```python
from build123d import *

# Parameters (mm, degrees)
F0_W     = 42.3
F0_H     = 42.3
F1_DEPTH = 48
F2_R     = 1.5
F3_DEPTH = 4.5
F4_R     = 11
F5_DEPTH = 2
F6_SIZE  = 5
F7_R     = 2.5
F8_DEPTH = 19
F9_R     = 0.5
F10_R    = 3


with BuildPart() as f1:
    # F0 (on Front) → F1 (new body)
    with BuildSketch(Plane.XZ):
        Rectangle(F0_W, F0_H)
    extrude(amount=F1_DEPTH)

    # F2 (on face) → F3 (cut)
    with BuildSketch(Plane.XZ.offset(48)):
        with Locations((-15.5, 15.5)):
            Circle(F2_R)
        with Locations((-15.5, -15.5)):
            Circle(F2_R)
        with Locations((15.5, -15.5)):
            Circle(F2_R)
        with Locations((15.5, 15.5)):
            Circle(F2_R)
    extrude(amount=-F3_DEPTH, mode=Mode.SUBTRACT)

    # F4 (on face) → F5 (join)
    with BuildSketch(Plane.XZ.offset(48)):
        Circle(F4_R)
    extrude(amount=F5_DEPTH)

    # F6
    f6_edges = [f1.edges().sort_by_distance(p)[0] for p in [
        (21.15, -24, 21.15),
        (-21.15, -24, 21.15),
        (-21.15, -24, -21.15),
        (21.15, -24, -21.15),
    ]]
    chamfer(f6_edges, length=F6_SIZE)

    # F7 (on face) → F8 (join)
    with BuildSketch(Plane.XZ.offset(50)):
        Circle(F7_R)
    extrude(amount=F8_DEPTH)

    # F9
    f9_edges = [f1.edges().sort_by_distance(p)[0] for p in [
        (-2.5, -69, 0),
    ]]
    fillet(f9_edges, radius=F9_R)

    # F10
    f10_edges = [f1.edges().sort_by_distance(p)[0] for p in [
        (16.15, -24, -21.15),
        (21.15, -24, -16.15),
        (-16.15, -24, -21.15),
        (-21.15, -24, -16.15),
        (21.15, -24, 16.15),
        (16.15, -24, 21.15),
        (-16.15, -24, 21.15),
        (-21.15, -24, 16.15),
    ]]
    fillet(f10_edges, radius=F10_R)


solid = f1.part
```
Design review of the part built by this model. Coordinates are the model's own, in mm. A direction names the side the tool comes from. Coordinates: 2 decimals unless noted, no trailing zeros. Write each loop counter-clockwise with the first axis right and the second up, starting at its lowest first coordinate (ties: lowest second). Pieces come first, ordered by that corner, then holes.
1) Mouldability with a two-part tool opening along Z and no side actions: class faces 1 (the cylindrical face through (-16.071, -24.336, 20.915)), 2 (the flat face through (15, -43.5, -15)), 3 (the flat face through (-3, -50, 0)), 4 (the cylindrical face through (-20.93, -24.34, -16.04)) as +Z half, -Z half, draft (parallel to the pull), parting line (faces both ways), or undercut.
2) Add section D-D (x = -4.5). Write out the cut boundary in (y, z), plus the area to 3 significant figures.
3) Insertion check: pin 1 (1 mm diameter, centred on x = 10.5, z = 3, fed in from -Y); pin 2 (0.9 mm diameter, centred on x = 16, z = -16, fed in from -Y); pin 3 (2.5 mm diameter, centred on x = -15, z = 16, fed in from -Y). Each pin has a flat end and moves straight along its axis. Give the tip position at first contact, or say it passes through.
4) Add section C-C (z = 5). Write out the cut boundary in (x, y).
5) Machinability: for faces 5 (the cylindrical face through (-17, -45.78, -15.43)), 6 (the cylindrical face through (-16.071, -24.336, -20.915)), which of the approach directions +Z, -Z, +X, -X, +Y, -Y give a long, thin tool a straight path to every point of the face, cutting with its end or side? Answer none if there is none.
6) Add section A-A (y = -14). Write out the cut boundary in (x, z).
7) Add section B-B (x = 0). Write out the cut boundary in (y, z).
8) To check wall thickness, follow L1, parallel to Z at x = -15.5, y = -47.1; L2, parallel to Z at x = 15, y = -46. State the ranges of each line that lie inside material, in increasing order.
Check result:
1. face 1: +Z half
1. face 2: undercut
1. face 3: draft
1. face 4: -Z half
2. outline: (-50, -10.04) - (-48, -10.04) - (-48, -21.15) - (0, -21.15) - (0, 21.15) - (-48, 21.15) - (-48, 10.04) - (-50, 10.04) - close
2. area: 2,070 mm2
3. pin 1: stops at y = -50
3. pin 2: stops at y = -43.5
3. pin 3: stops at y = -48
4. outline: (-21.15, -48) - (-9.8, -48) - (-9.8, -50) - (9.8, -50) - (9.8, -48) - (21.15, -48) - (21.15, 0) - (-21.15, 0) - close
5. face 5: -Y
5. face 6: -Z, -X, +Y, -Y
6. outline: (-21.15, -14.91) arc R3 ccw to (-20.27, -17.03) - (-17.03, -20.27) arc R3 ccw to (-14.91, -21.15) - (14.91, -21.15) arc R3 ccw to (17.03, -20.27) - (20.27, -17.03) arc R3 ccw to (21.15, -14.91) - (21.15, 14.91) arc R3 ccw to (20.27, 17.03) - (17.03, 20.27) arc R3 ccw to (14.91, 21.15) - (-14.91, 21.15) arc R3 ccw to (-17.03, 20.27) - (-20.27, 17.03) arc R3 ccw to (-21.15, 14.91) - close
7. outline: (-69, -2) arc R0.5 ccw to (-68.5, -2.5) - (-50, -2.5) - (-50, -11) - (-48, -11) - (-48, -21.15) - (0, -21.15) - (0, 21.15) - (-48, 21.15) - (-48, 11) - (-50, 11) - (-50, 2.5) - (-68.5, 2.5) arc R0.5 ccw to (-69, 2) - close
8. L1: z = -21.09 to -17, -14 to 14, 17 to 21.09
8. L2: z = -21.15 to -16.91, -14.09 to 14.09, 16.91 to 21.15
